CAD build for the part. Positions are in the model's coordinates, mm. Face numbers are marked on the shaded views. A direction names the side the tool comes from. Coordinates: 2 decimals unless noted, no trailing zeros. Order: outer loops, then holes, each group sorted by start corner. A loop starts at its lowest first (then second) coordinate and runs counter-clockwise, first axis right, second up. Notation, with made-up numbers: (-10.5, 16.5) -> (21.5, 16.5) arc R13 cw to (21.5, 24.5) -> close; hole circle Ø6 at (63, 49). An arc over 180 degrees is marked (long way). Use one line per item in the form item = value. Start each with the question number.
from build123d import *

# Parameters (mm, degrees)
ESQUISSE1_R             = 25
ESQUISSE1_R_2           = 2.1
ESQUISSE1_R_3           = 1.3
BOSS_EXTRU_1_DEPTH      = 2
ESQUISSE2_W             = 22
ESQUISSE2_H             = 10
ENL_V_MAT_EXTRU_1_DEPTH = 2
ESQUISSE3_R             = 2.8
ESQUISSE3_R_2           = 1.3
ESQUISSE3_R_3           = 4.6
ESQUISSE3_R_4           = 2.1
ESQUISSE3_R_5           = 3.6
BOSS_EXTRU_2_DEPTH      = 1
ESQUISSE4_OUTSIDE_W     = 66.154
ESQUISSE4_OUTSIDE_H     = 66.154
ENL_V_MAT_EXTRU_2_DEPTH = 4
CONG_1_R                = 2
ESQUISSE5_R             = 4.6
ESQUISSE5_R_2           = 2.1
BOSS_EXTRU_3_DEPTH      = 4
ESQUISSE6_R             = 30
ESQUISSE6_R_2           = 2.1
ESQUISSE6_R_3           = 1.3
BOSS_EXTRU_4_DEPTH      = 6
BOSS_EXTRU_4_DEPTH_BACK = 2
ESQUISSE7_R             = 2.1
ENL_V_MAT_EXTRU_3_DEPTH = 14
ESQUISSE8_R             = 3.6
ESQUISSE8_R_2           = 2.1
ENL_V_MAT_EXTRU_4_DEPTH = 3


with BuildPart() as part:
    # Esquisse1 → Boss.-Extru.1 (new body)
    with BuildSketch(Plane.XY):
        Circle(ESQUISSE1_R)
        with Locations((-14.142135624, 14.142135624)):
            Circle(ESQUISSE1_R_2, mode=Mode.SUBTRACT)
        with Locations((14.142135624, 14.142135624)):
            Circle(ESQUISSE1_R_2, mode=Mode.SUBTRACT)
        with Locations((-9, 5.5)):
            Circle(ESQUISSE1_R_3, mode=Mode.SUBTRACT)
        with Locations((-9, -5.5)):
            Circle(ESQUISSE1_R_3, mode=Mode.SUBTRACT)
        with Locations((9, 5.5)):
            Circle(ESQUISSE1_R_3, mode=Mode.SUBTRACT)
        with Locations((9, -5.5)):
            Circle(ESQUISSE1_R_3, mode=Mode.SUBTRACT)
    extrude(amount=BOSS_EXTRU_1_DEPTH)

    # Esquisse2 → Enlèv. mat.-Extru.1 (cut)
    with BuildSketch(Plane.XY.offset(2)):
        with Locations((0, -14)):
            Rectangle(ESQUISSE2_W, ESQUISSE2_H)
    extrude(amount=-ENL_V_MAT_EXTRU_1_DEPTH, mode=Mode.SUBTRACT)

    # Esquisse3 → Boss.-Extru.2 (add)
    with BuildSketch(Plane.XY.offset(2)):
        with Locations((-9, -5.5)):
            Circle(ESQUISSE3_R)
        with Locations((-9, -5.5)):
            Circle(ESQUISSE3_R_2, mode=Mode.SUBTRACT)
        with Locations((9, -5.5)):
            Circle(ESQUISSE3_R)
        with Locations((9, -5.5)):
            Circle(ESQUISSE3_R_2, mode=Mode.SUBTRACT)
        with Locations((9, 5.5)):
            Circle(ESQUISSE3_R)
        with Locations((9, 5.5)):
            Circle(ESQUISSE3_R_2, mode=Mode.SUBTRACT)
        with Locations((-9, 5.5)):
            Circle(ESQUISSE3_R)
        with Locations((-9, 5.5)):
            Circle(ESQUISSE3_R_2, mode=Mode.SUBTRACT)
        with Locations((-14.142135624, 14.142135624)):
            Circle(ESQUISSE3_R_3)
        with Locations((-14.142135624, 14.142135624)):
            Circle(ESQUISSE3_R_4, mode=Mode.SUBTRACT)
        with Locations((14.142135624, -14.142135624)):
            Circle(ESQUISSE3_R_5)
        with Locations((14.142135624, -14.142135624)):
            Circle(ESQUISSE3_R_4, mode=Mode.SUBTRACT)
        with Locations((-14.142135624, -14.142135624)):
            Circle(ESQUISSE3_R_5)
        with Locations((-14.142135624, -14.142135624)):
            Circle(ESQUISSE3_R_4, mode=Mode.SUBTRACT)
        with Locations((14.142135624, 14.142135624)):
            Circle(ESQUISSE3_R_3)
        with Locations((14.142135624, 14.142135624)):
            Circle(ESQUISSE3_R_4, mode=Mode.SUBTRACT)
    extrude(amount=BOSS_EXTRU_2_DEPTH)

    # Esquisse4 outside → Enlèv. mat.-Extru.2 (cut, through all)
    with BuildSketch(Plane(origin=(0, 0, 0), x_dir=(-1, 0, 0), z_dir=(0, 0, -1))):
        Rectangle(ESQUISSE4_OUTSIDE_W, ESQUISSE4_OUTSIDE_H)
        with BuildLine():
            Line((-14.142135624, 18.742135624), (14.142135624, 18.742135624))
            ThreePointArc((14.142135624, 18.742135624), (17.394826817, 17.394826817), (18.742135624, 14.142135624))
            Line((18.742135624, 14.142135624), (18.742135624, -9))
            Line((18.742135624, -9), (-18.742135624, -9))
            Line((-18.742135624, -9), (-18.742135624, 14.142135624))
            ThreePointArc((-18.742135624, 14.142135624), (-17.394826817, 17.394826817), (-14.142135624, 18.742135624))
        make_face(mode=Mode.SUBTRACT)
    extrude(amount=-ENL_V_MAT_EXTRU_2_DEPTH, mode=Mode.SUBTRACT)

    # Congé1
    cong_1_edges = [part.edges().sort_by_distance(p)[0] for p in [
        (-18.742135624, -9, 1),
        (18.742135624, -9, 1),
    ]]
    fillet(cong_1_edges, radius=CONG_1_R)

    # Esquisse5 → Boss.-Extru.3 (add)
    with BuildSketch(Plane.XY.offset(3)):
        with Locations((14.142135624, 14.142135624)):
            Circle(ESQUISSE5_R)
        with Locations((14.142135624, 14.142135624)):
            Circle(ESQUISSE5_R_2, mode=Mode.SUBTRACT)
        with Locations((-14.142135624, 14.142135624)):
            Circle(ESQUISSE5_R)
        with Locations((-14.142135624, 14.142135624)):
            Circle(ESQUISSE5_R_2, mode=Mode.SUBTRACT)
    extrude(amount=BOSS_EXTRU_3_DEPTH)

    # Esquisse6 → Boss.-Extru.4 (add, two sides)
    with BuildSketch(Plane(origin=(0, 0, 0), x_dir=(-1, 0, 0), z_dir=(0, 0, -1))) as boss_extru_4_sk:
        Circle(ESQUISSE6_R)
        with Locations((14.142135624, 14.142135624)):
            Circle(ESQUISSE6_R_2, mode=Mode.SUBTRACT)
        with Locations((9, 5.5)):
            Circle(ESQUISSE6_R_3, mode=Mode.SUBTRACT)
        with Locations((9, -5.5)):
            Circle(ESQUISSE6_R_3, mode=Mode.SUBTRACT)
        with Locations((-9, -5.5)):
            Circle(ESQUISSE6_R_3, mode=Mode.SUBTRACT)
        with Locations((-9, 5.5)):
            Circle(ESQUISSE6_R_3, mode=Mode.SUBTRACT)
        with Locations((-14.142135624, 14.142135624)):
            Circle(ESQUISSE6_R_2, mode=Mode.SUBTRACT)
    extrude(amount=BOSS_EXTRU_4_DEPTH)
    extrude(boss_extru_4_sk.sketch, amount=-BOSS_EXTRU_4_DEPTH_BACK)

    # Esquisse7 → Enlèv. mat.-Extru.3 (cut, through all)
    with BuildSketch(Plane(origin=(0, 0, -6), x_dir=(-1, 0, 0), z_dir=(0, 0, -1))):
        with Locations((-14.142135624, -14.142135624)):
            Circle(ESQUISSE7_R)
        with Locations((14.142135624, -14.142135624)):
            Circle(ESQUISSE7_R)
        with Locations((0, 25)):
            Circle(ESQUISSE7_R)
        with Locations((17.67766953, 17.67766953)):
            Circle(ESQUISSE7_R)
        with Locations((25, 0)):
            Circle(ESQUISSE7_R)
        with Locations((17.67766953, -17.67766953)):
            Circle(ESQUISSE7_R)
        with Locations((0, -25)):
            Circle(ESQUISSE7_R)
        with Locations((-17.67766953, -17.67766953)):
            Circle(ESQUISSE7_R)
        with Locations((-25, 0)):
            Circle(ESQUISSE7_R)
        with Locations((-17.67766953, 17.67766953)):
            Circle(ESQUISSE7_R)
    extrude(amount=-ENL_V_MAT_EXTRU_3_DEPTH, mode=Mode.SUBTRACT)

    # Esquisse8 → Enlèv. mat.-Extru.4 (cut)
    with BuildSketch(Plane(origin=(0, 0, -6), x_dir=(-1, 0, 0), z_dir=(0, 0, -1))):
        with Locations((-14.142135624, -14.142135624)):
            Circle(ESQUISSE8_R)
        with Locations((-14.142135624, -14.142135624)):
            Circle(ESQUISSE8_R_2, mode=Mode.SUBTRACT)
        with Locations((14.142135624, -14.142135624)):
            Circle(ESQUISSE8_R)
        with Locations((14.142135624, -14.142135624)):
            Circle(ESQUISSE8_R_2, mode=Mode.SUBTRACT)
        with Locations((14.142135624, 14.142135624)):
            Circle(ESQUISSE8_R)
        with Locations((14.142135624, 14.142135624)):
            Circle(ESQUISSE8_R_2, mode=Mode.SUBTRACT)
        with Locations((-14.142135624, 14.142135624)):
            Circle(ESQUISSE8_R)
        with Locations((-14.142135624, 14.142135624)):
            Circle(ESQUISSE8_R_2, mode=Mode.SUBTRACT)
    extrude(amount=-ENL_V_MAT_EXTRU_4_DEPTH, mode=Mode.SUBTRACT)


solid = part.part
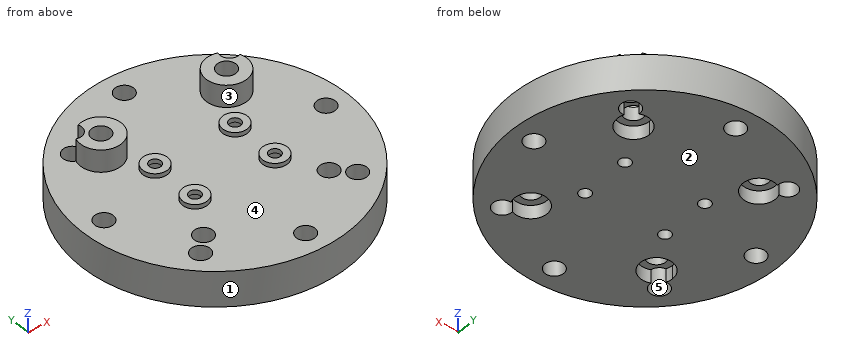
1) Cut at A-A on x = 0. Give the cut face in (y, z), then the cut area to 3 significant figures.
2) Cut at D-D on z = -4.5. Count the separate pieces of the cut face and the enclosed holes in it, then the cut area to 3 significant figures.
3) Cut at C-C on z = 5. Give the cut face in (x, y), then the cut area to 3 significant figures.
4) 3-axis set-ups, long thin cutter, end or side, ignore diameter. For the marked faces 4 and 5: which of +Z, -Z, +X, -X, +Y, -Y reach the whole face in a straight line?
5) Drop flat-ended pins along their axis: P1, Ø6.5, axis at x = 14.14, y = -14.14, coming from the +Z side; P2, Ø5, axis at y = 14, z = -4.5, coming from the +X side; P3, Ø4.5, axis at x = -8, y = 5.5, coming from the +Z side. Give the stop position or say it passes through.
6) Two-plate mould, pull along X, no slides. Class the marked faces 1, 2 and 3: released by +X, released by -X, zero draft, split by the parting line, or undercut.
7) Probe L1, parallel to Y at x = 9, z = 2.3; L2, parallel to X at y = -6, z = -1; L3, parallel to Y at x = -19.5, z = -4.75. List the from-to ranges inside material, lowest first.
Values follow:
q1.outline = (-30, -6) -> (-27.1, -6) -> (-27.1, 2) -> (-30, 2) -> close; (-22.9, -6) -> (22.9, -6) -> (22.9, 2) -> (-22.9, 2) -> close; (27.1, -6) -> (30, -6) -> (30, 2) -> (27.1, 2) -> close
q1.area = 413 mm^2
q2.separate_pieces = 1
q2.enclosed_holes = 12
q2.area = 2,540 mm^2
q3.outline = (-18.46, 15.73) arc R4.6 ccw (long way) to (-15.73, 18.46) arc R2.1 cw to start; (15.73, 18.46) arc R4.6 ccw (long way) to (18.46, 15.73) arc R2.1 cw to start; hole circle Ø4.2 at (-14.14, 14.14); hole circle Ø4.2 at (14.14, 14.14)
q3.area = 95.9 mm^2
q4.face_4 = +Z
q4.face_5 = +Z, -Z
q5.P1 = 2
q5.P2 = 27.71
q5.P3 = 3
q6.face_1 = split by the parting line
q6.face_2 = zero draft
q6.face_3 = undercut
q7.L1 = -8.3 to -6.8, -4.2 to -2.7, 2.7 to 4.2, 6.8 to 8.3
q7.L2 = -29.39 to -10.2, -7.8 to 7.8, 10.2 to 29.39
q7.L3 = -22.8 to -18.72, -16.63 to 16.63, 18.72 to 22.8
